from build123d import *

# Parameters (mm, degrees)
SKETCH_1_R          = 5.5
EXTRUDE_1_DEPTH     = 15
SKETCH_3_R          = 7.159544481
CUT_EXTRUDE_1_DEPTH = 7


with BuildPart() as part:
    # 스케치1 → 보스-돌출1 (new body)
    with BuildSketch(Plane.XY):
        Circle(SKETCH_1_R)
    extrude(amount=EXTRUDE_1_DEPTH)

    # 스케치2 → 회전1 (revolve)
    with BuildSketch(Plane(origin=(0, 0, 0), x_dir=(1, 0, 0), z_dir=(0, 1, 0)), mode=Mode.PRIVATE) as revolve_1_sk:
        with BuildLine():
            Line((0, 18.371801754), (0, 0))
            Line((0, 0), (-5.469271925, 0))
            ThreePointArc((-5.469271925, 0), (-9.584310553, 11.225043985), (0, 18.371801754))
        make_face()
    revolve(revolve_1_sk.sketch.rotate(Axis((0, 0, -18.371801754), (0, 0, 1)), 180), axis=Axis((0, 0, -18.371801754), (0, 0, 1)))

    # 스케치3 → 컷-돌출1 (cut)
    with BuildSketch(Plane.XY.offset(15)):
        Circle(SKETCH_3_R)
    extrude(amount=-CUT_EXTRUDE_1_DEPTH, mode=Mode.SUBTRACT)


solid = part.part
Verification items for the finished model (mm, model axes). A direction names the side the tool comes from. Give positions to 0.01 mm unless a question says otherwise; leave off trailing zeros. Order: outer loops, then holes, each group sorted by start corner. A loop starts at its lowest first (then second) coordinate and runs counter-clockwise, first axis right, second up. Notation, with made-up numbers: M 45,11.5 L 100,11.5 A27 ccw 100,39.5 Z; hole C 85,-14 d1. An arc over 180 degrees is marked long. Answer as a JSON object with one key per item and string values. Group by question number.
1) Cross-section at B-B (z = 3.75). Enter the section's corners in (x, y).
2) Depth check by flat-ended pin: pin 1 Ø1.5 at (x, z) = (1, 4) entering from +Y; pin 2 Ø8 at (y, z) = (-5, 0.5) entering from +X; pin 3 Ø6 at (x, z) = (-7, -8) entering from +Y. Enter the tip coordinate at first touch or a pass-through.
3) Scan lines: line 1 along Y through (x, z) = (-0.25, 4); line 2 along Z through (x, y) = (-1.25, -4.25); line 3 along Y through (x, z) = (2.75, -14). Record each from-to range of solid material in increasing order. Write a range as [from, to].
4) Access from +Z, -Z, +X, -X, +Y, -Y to the whole of each face (thin tool, end or side, straight path). Record for faces 1 (the face through (-1.19, -5.37, 3.94)), 2 (the face through (0, 0, 8)).
5) Cross-section at D-D (x = 8.75). Enter the section's corners in (y, z).
Result sheet:
{
 "1": {"outline": "C 0,0 d11"},
 "2": {"pin 1": "stops at y = 5.49", "pin 2": "stops at x = 7.86", "pin 3": "stops at y = 9.16"},
 "3": {"line 1": "y = [-5.49, 5.49]", "line 2": "z = [-17.34, 8]", "line 3": "y = [-7.79, 7.79]"},
 "4": {"face 1": "+Z", "face 2": "+Z, +X, -X, +Y, -Y"},
 "5": {"outline": "C 0,-8.37 d9.68"}
}
